Could you check a few things on this model? Use its own coordinates, in mm. Face numbers are marked on the shaded views. A direction names the side the tool comes from. Round coordinates to 2 decimals unless told otherwise and drop trailing zeros. Write each loop counter-clockwise with the first axis right and the second up, starting at its lowest first coordinate (ties: lowest second). Pieces come first, ordered by that corner, then holes. Notation, with made-up numbers: (9.5, 34.5) - (65.5, 34.5) arc R20 ccw to (65.5, 66.5) - close; hole circle Ø4 at (38, -25.75). An arc over 180 degrees is marked (long way). Write each question's results on one line, items separated by ' | '. Start each with the question number.
(1) Imagine slicing it at C-C on x = -27. Write out the boundary of the cut face in (y, z).
(2) Imagine slicing it at A-A on y = 11.5. Write out the boundary of the cut face in (x, z).
(3) Imagine slicing it at D-D on z = -1.5. Write out the boundary of the cut face in (x, y).
(4) On a 3-axis mill with a long thin cutter (end or side, diameter ignored), from which of +Z, -Z, +X, -X, +Y, -Y can I reach the whole of each face in a straight line? I mean the marked faces 4, 5 and 6. Say none if no direction works.
(5) Imagine slicing it at B-B on z = -3.95. Write out the boundary of the cut face in (x, y).
(6) Thinking about a two-plate mould opening in Y: for the marked faces 1, 2 and 3, which applies, +Y half, -Y half, draft (parallel to the pull), parting line (faces both ways), or undercut?
(7) For P1, Ø1, axis at x = -13.5, z = -2.5, coming from the -Y side; P2, Ø4, axis at x = -8.5, z = -5.5, coming from the +Y side; P3, Ø1, axis at x = -17, z = -1.5, coming from the -Y side; P4, Ø2.5, axis at x = -27, z = -3.95, coming from the +Y side, each with a flat end and sliding along its axis, tell me the tip position at first contact or that it passes through.
(8) Please list where these lines run through material, in increasing order: line 1 (Y direction, x = -25.5, z = -3.25); line 2 (Z direction, x = -27, y = 16.75); line 3 (X direction, y = 4.5, z = -6). Write a range as [from, to].
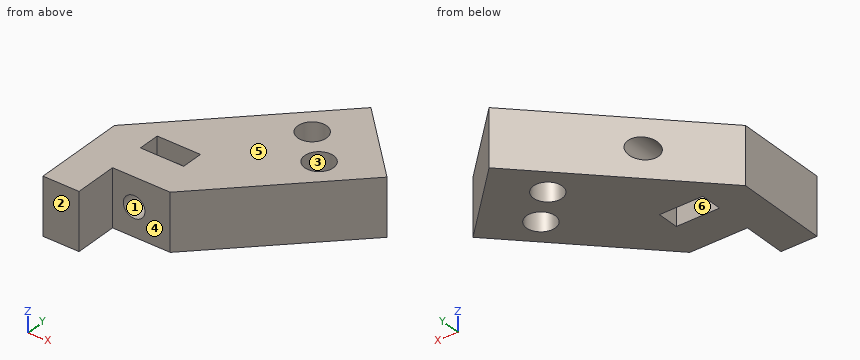
```python
from build123d import *

# Parameters (mm, degrees)
SKETCH1_R           = 2
BOSS_EXTRUDE1_DEPTH = 7.9
SKETCH2_R           = 1.5
CUT_EXTRUDE1_DEPTH  = 45.813969002
SKETCH3_W           = 6
SKETCH3_H           = 3
CUT_EXTRUDE2_DEPTH  = 49.646507856


with BuildPart() as part:
    # Sketch1 → Boss-Extrude1 (new body)
    with BuildSketch(Plane.XY):
        Polygon((-30, 0), (-30, 6), (-22, 6), (-5.050252532, 22.949747468), (-14.949747468, 32.849242405), (-35, 12.798989873), (-35, 0), align=None)
        with Locations((-12.828427125, 20.828427125)):
            Circle(SKETCH1_R, mode=Mode.SUBTRACT)
        with Locations((-17.071067812, 25.071067812)):
            Circle(SKETCH1_R, mode=Mode.SUBTRACT)
    extrude(amount=-BOSS_EXTRUDE1_DEPTH)

    # Sketch2 → Cut-Extrude1 (cut, through all)
    with BuildSketch(Plane.XZ.offset(-6)):
        with Locations(Location((-27, -3.95, 0), (0, 0, 270))):
            Circle(SKETCH2_R)
    extrude(amount=-CUT_EXTRUDE1_DEPTH, mode=Mode.SUBTRACT)

    # Sketch3 → Cut-Extrude2 (cut, through all)
    with BuildSketch(Plane.XY):
        with Locations((-27, 12.5)):
            Rectangle(SKETCH3_W, SKETCH3_H)
    extrude(amount=-CUT_EXTRUDE2_DEPTH, mode=Mode.SUBTRACT)


solid = part.part
```
Response:
1) outline: (6, -7.9) - (11, -7.9) - (11, -5.45) - (6, -5.45) - close; (6, -2.45) - (11, -2.45) - (11, 0) - (6, 0) - close; (14, -7.9) - (20.8, -7.9) - (20.8, -5.45) - (14, -5.45) - close; (14, -2.45) - (20.8, -2.45) - (20.8, 0) - (14, 0) - close
2) outline: (-35, -7.9) - (-30, -7.9) - (-30, 0) - (-35, 0) - close; (-24, -7.9) - (-16.5, -7.9) - (-16.5, 0) - (-24, 0) - close
3) outline: (-35, 0) - (-30, 0) - (-30, 6) - (-22, 6) - (-5.05, 22.95) - (-14.95, 32.85) - (-35, 12.8) - close; hole (-30, 11) - (-24, 11) - (-24, 14) - (-30, 14) - close; hole circle Ø4 at (-17.07, 25.07); hole circle Ø4 at (-12.83, 20.83)
4) face 4: +Z, -Z, +X, -Y | face 5: +Z, +X, -X, +Y, -Y | face 6: +Z, -Z
5) outline: (-35, 0) - (-30, 0) - (-30, 6) - (-28.5, 6) - (-28.5, 11) - (-30, 11) - (-30, 14) - (-28.5, 14) - (-28.5, 19.3) - (-35, 12.8) - close; (-25.5, 6) - (-22, 6) - (-5.05, 22.95) - (-14.95, 32.85) - (-25.5, 22.3) - (-25.5, 14) - (-24, 14) - (-24, 11) - (-25.5, 11) - close; hole circle Ø4 at (-17.07, 25.07); hole circle Ø4 at (-12.83, 20.83)
6) face 1: draft | face 2: -Y half | face 3: undercut
7) P1: y = 14 | P2: y = 28.4 | P3: y = 10.5 | P4: through
8) line 1: [6, 11], [14, 22.3] | line 2: [-7.9, -5.45], [-2.45, 0] | line 3: [-35, -30]
